from build123d import *

# Parameters (mm, degrees)
SKETCH1_R           = 27.1
SKETCH1_R_2         = 5
BOSS_EXTRUDE1_DEPTH = 100
CUT_EXTRUDE1_START  = -7.15
SKETCH2_R           = 7
SKETCH2_R_2         = 5
CUT_EXTRUDE1_DEPTH  = 7.15
CUT_EXTRUDE2_START  = -8
SKETCH3_R           = 11.25
SKETCH3_R_2         = 7
CUT_EXTRUDE2_DEPTH  = 8
SKETCH4_R           = 7
CUT_EXTRUDE3_DEPTH  = 7.15
SKETCH5_R           = 11.25
SKETCH5_R_2         = 7
CUT_EXTRUDE4_DEPTH  = 8


with BuildPart() as part:
    # Sketch1 → Boss-Extrude1 (new body)
    with BuildSketch(Plane.XY):
        Circle(SKETCH1_R)
        Circle(SKETCH1_R_2, mode=Mode.SUBTRACT)
    extrude(amount=BOSS_EXTRUDE1_DEPTH)

    # Sketch2 → Cut-Extrude1 (cut)
    with BuildSketch(Plane.XY.offset(100).offset(CUT_EXTRUDE1_START)):
        Circle(SKETCH2_R)
        Circle(SKETCH2_R_2, mode=Mode.SUBTRACT)
    extrude(amount=CUT_EXTRUDE1_DEPTH, mode=Mode.SUBTRACT)

    # Sketch3 → Cut-Extrude2 (cut)
    with BuildSketch(Plane.XY.offset(100).offset(CUT_EXTRUDE2_START)):
        Circle(SKETCH3_R)
        Circle(SKETCH3_R_2, mode=Mode.SUBTRACT)
    extrude(amount=CUT_EXTRUDE2_DEPTH, mode=Mode.SUBTRACT)

    # Sketch4 → Cut-Extrude3 (cut)
    with BuildSketch(Plane(origin=(0, 0, 0), x_dir=(-1, 0, 0), z_dir=(0, 0, -1))):
        with Locations(Location((0, 0, 0), (0, 0, 180))):
            Circle(SKETCH4_R)
    extrude(amount=-CUT_EXTRUDE3_DEPTH, mode=Mode.SUBTRACT)

    # Sketch5 → Cut-Extrude4 (cut)
    with BuildSketch(Plane(origin=(0, 0, 0), x_dir=(-1, 0, 0), z_dir=(0, 0, -1))):
        with Locations(Location((0, 0, 0), (0, 0, 180))):
            Circle(SKETCH5_R)
        with Locations(Location((0, 0, 0), (0, 0, 180))):
            Circle(SKETCH5_R_2, mode=Mode.SUBTRACT)
    extrude(amount=-CUT_EXTRUDE4_DEPTH, mode=Mode.SUBTRACT)


solid = part.part
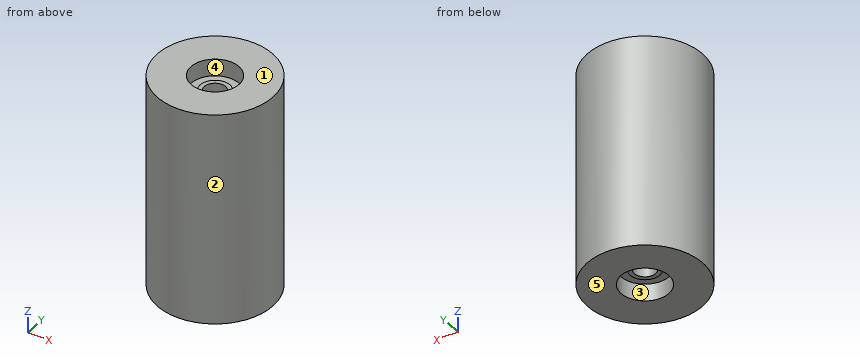
The listing builds one solid part. Answer for the finished solid, in the listing's coordinates (mm). Face numbers are marked on the shaded views. A direction names the side the tool comes from. Give positions to 0.01 mm unless a question says otherwise; leave off trailing zeros. Loops run counter-clockwise (first coordinate to the right, second up) from the corner with the lowest first, then second, coordinate; pieces in that order, holes last. Notation, with made-up numbers: (-12, 46.5) - (0, 46.5) arc R29 ccw to (0, 68.5) - close; hole circle Ø11 at (77.5, 12.5). An arc over 180 degrees is marked (long way). Answer as a JSON object with one key per item and string values.
1. A cutting plane is placed at C-C (z = 44.5). Write down the section's boundary in (x, y), then the cut area to 3 significant figures.
Determined:
{"outline": "circle Ø54.2 at (0, 0); hole circle Ø10 at (0, 0)", "area": "2,230 mm²"}
2. A cutting plane is placed at D-D (y = -20.5). Write down the section's boundary in (x, z), then the cut area to 3 significant figures.
Determined:
{"outline": "(-17.72, 0) - (17.72, 0) - (17.72, 100) - (-17.72, 100) - close", "area": "3,540 mm²"}
3. Flat-ended cylindrical pins translate along their axes: pin 1 Ø4 at (x, y) = (0.5, -3) entering from -Z; pin 2 Ø15.5 at (x, y) = (-2.5, -1) entering from +Z; pin 3 Ø25 at (x, y) = (-1, -1) entering from +Z; pin 4 Ø8 at (x, z) = (-17, 14.5) entering from +Y. Find the tip coordinate at first contact, or state that the pin passes through.
Determined:
{"pin 1": "z = 7.15", "pin 2": "z = 92.85", "pin 3": "z = 100", "pin 4": "y = 23.78"}
4. For a pull along X with two mould halves and no side action, classify the marked faces 1, 2 and 3 as pulls with the +X half, pulls with the -X half, needs draft (parallel to the pull), parting line crosses it, or undercut.
Determined:
{"face 1": "needs draft", "face 2": "parting line crosses it", "face 3": "undercut"}
5. For the marked faces 4 and 5, determine the directions among +Z, -Z, +X, -X, +Y, -Y from which every point of the face is accessible in a straight line to the end or side of a thin tool.
Determined:
{"face 4": "+Z", "face 5": "-Z, +X, -X, +Y, -Y"}
6. A cutting plane is placed at A-A (y = 0). Write down the section's boundary in (x, z), then the cut area to 3 significant figures.
Determined:
{"outline": "(-27.1, 0) - (-11.25, 0) - (-11.25, 8) - (-7, 8) - (-7, 7.15) - (-5, 7.15) - (-5, 92.85) - (-7, 92.85) - (-7, 92) - (-11.25, 92) - (-11.25, 100) - (-27.1, 100) - close; (5, 7.15) - (7, 7.15) - (7, 8) - (11.25, 8) - (11.25, 0) - (27.1, 0) - (27.1, 100) - (11.25, 100) - (11.25, 92) - (7, 92) - (7, 92.85) - (5, 92.85) - close", "area": "4,230 mm²"}
7. Find the intervals of material crossed by L1, parallel to Y at x = 0, z = 98; L2, parallel to Z at x = 0, y = 8; L3, parallel to X at y = 0.5, z = 13.5, in increasing order. Write a range as [from, to].
Determined:
{"L1": "[-27.1, -11.25], [11.25, 27.1]", "L2": "[8, 92]", "L3": "[-27.1, -4.97], [4.97, 27.1]"}
